Job drawing, mm, ordinate dimensions from the low corner. One solid piece. Round coordinates to 2 decimals unless told otherwise and drop trailing zeros. Loops run counter-clockwise (first coordinate to the right, second up) from the corner with the lowest first, then second, coordinate; pieces in that order, holes last. Notation, with made-up numbers: (-12.5, -10) - (35.5, -10) arc R28 cw to (35.5, 24) - close; hole circle Ø9 at (-10.5, -25). An arc over 180 degrees is marked (long way). Answer as CSV lines item,"result". Start each with the question number.
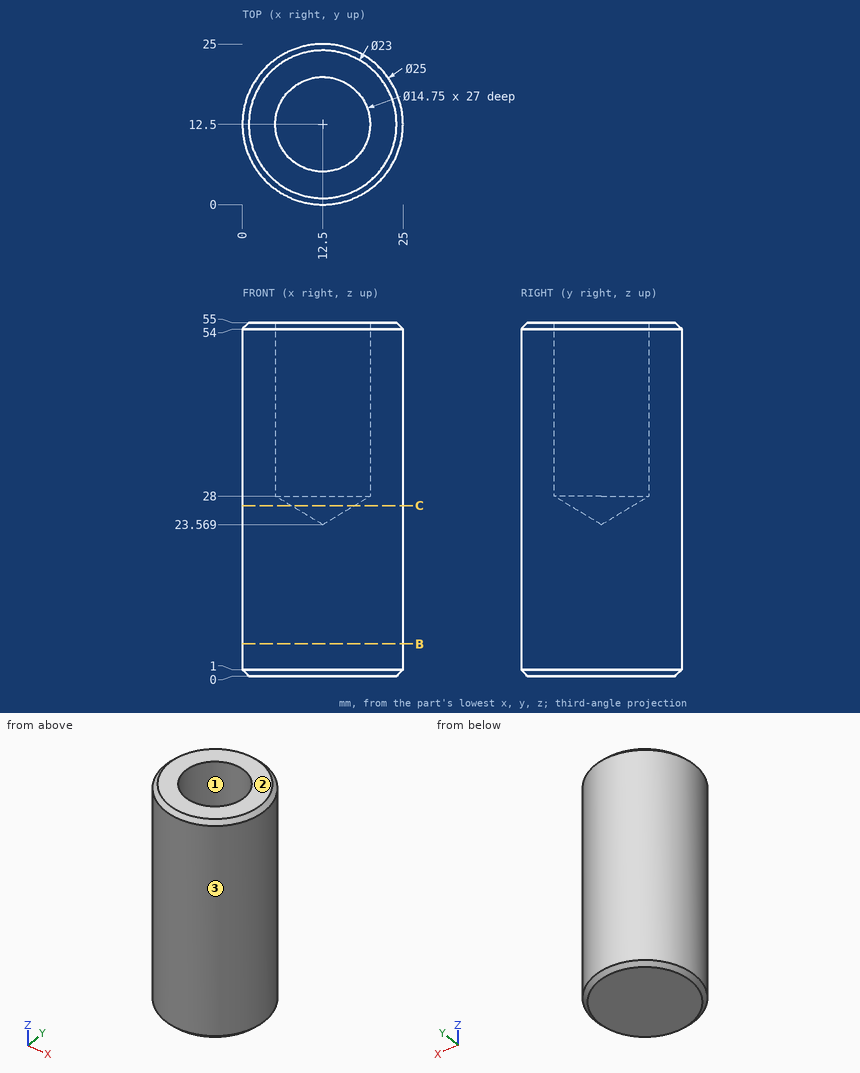
Q1. Pin check, flat tips, straight feed: pin 1 Ø3 at (y, z) = (2.5, 37.5) entering from -X (1 decimal); pin 2 Ø1 at (y, z) = (10, 25) entering from -X; pin 3 Ø4 at (x, z) = (8.5, 33.5) entering from +Y. Stop position of each tip, or through.
Q2. Band-saw the part on C-C, the plane z = 26.5. List the corners of the cut face in (x, y).
Q3. Band-saw the part on B-B, the plane z = 5. List the corners of the cut face in (x, y).
Q4. Two-plate mould, pull along Y, no slides. Class the marked faces 1, 2 and 3: released by +Y, released by -Y, zero draft, split by the parting line, or undercut.
Q5. Wall check: probe 1 along Y at (x, z) = (12.5, 34.5) (1 decimal); probe 2 along Y at (x, z) = (6.75, 30.5); probe 3 along X at (y, z) = (17, 50.5). Give the ranges that are in metal, low to high. Write a range as [from, to].
Reported:
1,pin 1,"stops at x = 3.3"
1,pin 2,"stops at x = 0.16"
1,pin 3,"stops at y = 24.84"
2,outline,"circle Ø25 at (12.5, 12.5); hole circle Ø9.76 at (12.5, 12.5)"
3,outline,"circle Ø25 at (12.5, 12.5)"
4,face 1,"undercut"
4,face 2,"zero draft"
4,face 3,"split by the parting line"
5,probe 1,"y = [0, 5.1], [19.9, 25]"
5,probe 2,"y = [1.4, 7.88], [17.12, 23.6]"
5,probe 3,"x = [0.84, 6.66], [18.34, 24.16]"
